```python
from build123d import *

# Parameters (mm, degrees)
F1_DEPTH = 232.2576
F2_W     = 308.927283
F2_H     = 195.242041
F3_DEPTH = 91.44
F5_DEPTH = 508


with BuildPart() as f1:
    # F0 (on Top) → F1 (new body)
    with BuildSketch(Plane.XY):
        with BuildLine():
            ThreePointArc((-173.357227, 18.40329), (-1.055729, 114.038895), (173.772714, 23.104903))
            ThreePointArc((173.772714, 23.104903), (-1.064562, 114.691102), (-173.357227, 18.40329))
        make_face()
        with BuildLine():
            Line((173.772714, -51.430393), (173.772714, 23.104903))
            ThreePointArc((173.772714, 23.104903), (-1.055729, 114.038895), (-173.357227, 18.40329))
            Line((-173.357227, 18.40329), (-173.357227, -51.430393))
            Line((-173.357227, -51.430393), (173.772714, -51.430393))
        make_face()
    extrude(amount=F1_DEPTH)

    # F2 (on face) → F3 (cut)
    with BuildSketch(Plane.XZ.offset(51.430393)):
        with Locations((0.790856, 109.876665)):
            Rectangle(F2_W, F2_H)
    extrude(amount=-F3_DEPTH, mode=Mode.SUBTRACT)

    # F4 (on face) → F5 (cut)
    with BuildSketch(Plane.XY.offset(232.2576)):
        Polygon((-128.352299, 26.706169), (-128.352299, -6.949546), (-110.229991, -17.952379), (-85.635431, -6.949546), (-85.635431, 26.706169), (-110.229991, 38.356224), align=None)
        Polygon((-52.128345, 6.618178), (-52.128345, -27.037537), (-34.006037, -38.04037), (-9.411477, -27.037537), (-9.411477, 6.618178), (-34.006037, 18.268233), align=None)
        Polygon((17.95378, 9.17491), (17.95378, -24.480805), (36.076088, -35.483638), (60.670648, -24.480805), (60.670648, 9.17491), (36.076088, 20.824965), align=None)
        Polygon((113.401607, 9.17491), (113.401607, -24.480805), (131.523915, -35.483638), (156.118475, -24.480805), (156.118475, 9.17491), (131.523915, 20.824965), align=None)
        Polygon((70.684742, 71.302582), (70.684742, 37.646867), (88.80705, 26.644034), (113.40161, 37.646867), (113.40161, 71.302582), (88.80705, 82.952637), align=None)
        Polygon((-40.650681, 82.305415), (-40.650681, 48.6497), (-22.528373, 37.646867), (2.066188, 48.6497), (2.066188, 82.305415), (-22.528373, 93.95547), align=None)
    extrude(amount=-F5_DEPTH, mode=Mode.SUBTRACT)


solid = f1.part
```
CAD build for the part. Positions are in the model's coordinates, mm. A direction names the side the tool comes from. Round coordinates to 2 decimals unless told otherwise and drop trailing zeros. Loops run counter-clockwise (first coordinate to the right, second up) from the corner with the lowest first, then second, coordinate; pieces in that order, holes last. Notation, with made-up numbers: (33, 86.25) - (45, 86.25) arc R29 cw to (45, 108.25) - close; hole circle Ø3 at (63.5, -22.75). An arc over 180 degrees is marked (long way). Return JSON: item names as keys, results as strings. Group by question number.
Q1. Band-saw the part on C-C on y = 87. Give the cut face in (x, z).
Q2. Band-saw the part on B-B on x = -114.5. Give the cut face in (y, z), plus the area to 3 significant figures.
Q3. Drill centre lines: line 1 along X through (y, z) = (3, 221); line 2 along X through (y, z) = (-36, 175.5); line 3 along Z through (x, y) = (136.5, 37.5). Where is each one in solid material? Low to high. Write a range as [from, to].
Q4. Two-plate mould, pull along X, no slides. Class faces 1 (the face through (-2, 33, 0)), 2 (the face through (1.82, 114.71, 114.5)), 3 (the face through (-85.635, 10, 6)): +X half, -X half, draft (parallel to the pull), parting line (faces both ways), or undercut.
Q5. Band-saw the part on D-D on x = -3. Give the cut face in (y, z).
Q6. Flat gauge pins, fed straight in: pin 1 Ø1.5 at (x, z) = (-130.5, 175) entering from +Y; pin 2 Ø10 at (y, z) = (73.5, 162) entering from +X; pin 3 Ø6 at (x, z) = (86, 131) entering from +Y. Where does each tip first touch, or does it go through?
Q7. Tool access for faces 4 (the face through (48.2, -30.06, 220.05)), 5 (the face through (-173.357, -16, 115)), 6 (the face through (26, 40.01, 111)): list every direction of +Z, -Z, +X, -X, +Y, -Y with a clear straight run to the whole face (end or side of a thin tool).
Q8. Band-saw the part on A-A on z = 59.5. Give the cut face in (x, y), plus the area to 3 significant figures.
Solutions:
{
 "1": {"outline": "(-101.81, 0) - (-33.35, 0) - (-33.35, 232.26) - (-101.81, 232.26) - close; (-7.84, 0) - (105.29, 0) - (105.29, 232.26) - (-7.84, 232.26) - close"},
 "2": {"outline": "(-51.43, 0) - (-15.36, 0) - (-15.36, 12.26) - (-51.43, 12.26) - close; (-51.43, 207.5) - (-15.36, 207.5) - (-15.36, 232.26) - (-51.43, 232.26) - close; (35.61, 0) - (79.06, 0) - (79.06, 232.26) - (35.61, 232.26) - (35.61, 207.5) - (40.01, 207.5) - (40.01, 12.26) - (35.61, 12.26) - close", "area": "10,600 mm^2"},
 "3": {"line 1": "x = [-173.36, -128.35], [-85.64, -52.13], [-9.41, 17.95], [60.67, 113.4], [156.12, 173.77]", "line 2": "x = [-173.36, -153.67], [155.25, 173.77]", "line 3": "z = [0, 12.26], [207.5, 232.26]"},
 "4": {"face 1": "draft", "face 2": "parting line", "face 3": "undercut"},
 "5": {"outline": "(-51.43, 0) - (46.38, 0) - (46.38, 232.26) - (-51.43, 232.26) - (-51.43, 207.5) - (40.01, 207.5) - (40.01, 12.26) - (-51.43, 12.26) - close; (84.71, 0) - (114.66, 0) - (114.66, 232.26) - (84.71, 232.26) - close"},
 "6": {"pin 1": "stops at y = 67.68", "pin 2": "stops at x = 132.23", "pin 3": "stops at y = 98.12"},
 "7": {"face 4": "+Z, -Z", "face 5": "+Z, -Z, -X, +Y, -Y", "face 6": "-Y"},
 "8": {"outline": "(-173.36, -51.43) - (-153.67, -51.43) - (-153.67, 40.01) - (-26.42, 40.01) - (-40.65, 48.65) - (-40.65, 82.31) - (-22.53, 93.96) - (2.07, 82.31) - (2.07, 48.65) - (-17.25, 40.01) - (70.68, 40.01) - (70.68, 71.3) - (88.81, 82.95) - (113.4, 71.3) - (113.4, 40.01) - (155.25, 40.01) - (155.25, 9.58) - (156.12, 9.17) - (156.12, -24.48) - (155.25, -24.87) - (155.25, -51.43) - (173.77, -51.43) - (173.77, 23.1) arc R207.33 ccw to (-173.36, 18.4) - close", "area": "16,300 mm^2"}
}
